Geometry: final body of the model. Coordinates: model frame, mm. A direction names the side the tool comes from. Coordinates: 2 decimals unless noted, no trailing zeros. Loops run counter-clockwise (first coordinate to the right, second up) from the corner with the lowest first, then second, coordinate; pieces in that order, holes last. Notation, with made-up numbers: (-21.5, 36) - (-7.5, 36) arc R20 ccw to (-7.5, 58) - close; hole circle Ø6 at (81.5, -3.75). An arc over 180 degrees is marked (long way). Answer in a Markdown table with one row per item.
from build123d import *

# Parameters (mm, degrees)
SKETCH1_W           = 101.6
SKETCH1_H           = 152.4
BOSS_EXTRUDE1_DEPTH = 3.175
SKETCH2_W           = 3.175
SKETCH2_H           = 12.7
CUT_EXTRUDE1_DEPTH  = 3.175
LPATTERN1_COUNT     = 5
LPATTERN1_PITCH     = 25.4
SKETCH3_W           = 3.175
SKETCH3_H           = 12.7
CUT_EXTRUDE2_DEPTH  = 3.175
LPATTERN2_COUNT     = 4
LPATTERN2_PITCH     = 25.4
SKETCH5_W           = 3.175
SKETCH5_H           = 57.15
CUT_EXTRUDE3_DEPTH  = 3.175
FILLET1_R           = 1.524
BOSS_EXTRUDE2_DEPTH = 3.175
SKETCH7_W           = 25.4
SKETCH7_H           = 95.25
CUT_EXTRUDE4_DEPTH  = 3.175
FILLET2_R           = 12.7


with BuildPart() as part:
    # Sketch1 → Boss-Extrude1 (new body)
    with BuildSketch(Plane(origin=(0, 0, 0), x_dir=(1, 0, 0), z_dir=(0, 1, 0))):
        with Locations((50.8, 76.2)):
            Rectangle(SKETCH1_W, SKETCH1_H)
        Polygon((0, 0), (101.6, -17.91482124), (101.6, 0), align=None)
    extrude(amount=BOSS_EXTRUDE1_DEPTH)

    # Sketch2 → Cut-Extrude1 (cut)
    with BuildSketch(Plane(origin=(0, 3.175, 0), x_dir=(1, 0, 0), z_dir=(0, 1, 0))):
        with Locations((1.5875, 133.35)):
            Rectangle(SKETCH2_W, SKETCH2_H)
    cut_extrude1 = extrude(amount=-CUT_EXTRUDE1_DEPTH, mode=Mode.SUBTRACT)

    # LPattern1: Cut-Extrude1 ×5
    with Locations(*[(0, 0, i * LPATTERN1_PITCH) for i in range(1, LPATTERN1_COUNT)]):
        add(cut_extrude1, mode=Mode.SUBTRACT)

    # Sketch3 → Cut-Extrude2 (cut)
    with BuildSketch(Plane(origin=(0, 3.175, 0), x_dir=(1, 0, 0), z_dir=(0, 1, 0))):
        with Locations((74.6125, 133.35)):
            Rectangle(SKETCH3_W, SKETCH3_H)
    cut_extrude2 = extrude(amount=-CUT_EXTRUDE2_DEPTH, mode=Mode.SUBTRACT)

    # LPattern2: Cut-Extrude2 ×4
    with Locations(*[(0, 0, i * LPATTERN2_PITCH) for i in range(1, LPATTERN2_COUNT)]):
        add(cut_extrude2, mode=Mode.SUBTRACT)

    # Sketch5 → Cut-Extrude3 (cut)
    with BuildSketch(Plane(origin=(0, 3.175, 0), x_dir=(1, 0, 0), z_dir=(0, 1, 0))):
        with Locations((33.3375, 10.66017876)):
            Rectangle(SKETCH5_W, SKETCH5_H)
        with Locations((90.4875, 10.66017876)):
            Rectangle(SKETCH5_W, SKETCH5_H)
    extrude(amount=-CUT_EXTRUDE3_DEPTH, mode=Mode.SUBTRACT)

    # Fillet1
    fillet1_edges = [part.edges().sort_by_distance(p)[0] for p in [
        (34.925, 1.5875, -39.23517876),
        (31.75, 1.5875, -39.23517876),
        (92.075, 1.5875, -39.23517876),
        (88.9, 1.5875, -39.23517876),
    ]]
    fillet(fillet1_edges, radius=FILLET1_R)

    # Sketch6 → Boss-Extrude2 (add)
    with BuildSketch(Plane(origin=(0, 3.175, 0), x_dir=(1, 0, 0), z_dir=(0, 1, 0))):
        Polygon((34.925, -6.158219801), (43.30472917, -7.635792145), (42.753396206, -10.762556761), (34.373667036, -9.284984417), align=None)
        Polygon((55.811787634, -9.841124001), (80.82590456, -14.251787714), (80.274571596, -17.37855233), (55.26045467, -12.967888617), align=None)
    extrude(amount=-BOSS_EXTRUDE2_DEPTH)

    # Sketch7 → Cut-Extrude4 (cut)
    with BuildSketch(Plane(origin=(0, 3.175, 0), x_dir=(1, 0, 0), z_dir=(0, 1, 0))):
        with Locations((22.225, 98.425)):
            Rectangle(SKETCH7_W, SKETCH7_H)
        with Locations((53.975, 98.425)):
            Rectangle(SKETCH7_W, SKETCH7_H)
    extrude(amount=-CUT_EXTRUDE4_DEPTH, mode=Mode.SUBTRACT)

    # Fillet2
    fillet2_edges = [part.edges().sort_by_distance(p)[0] for p in [
        (66.675, 1.5875, -146.05),
        (34.925, 1.5875, -146.05),
        (41.275, 1.5875, -146.05),
        (9.525, 1.5875, -146.05),
        (34.925, 1.5875, -50.8),
        (41.275, 1.5875, -50.8),
        (66.675, 1.5875, -50.8),
        (9.525, 1.5875, -50.8),
    ]]
    fillet(fillet2_edges, radius=FILLET2_R - 0.0001)  # a hair under: the kernel refuses the full size


solid = part.part
(1) Cut plane C-C on z = -70. Output: boundary loops of the cut face in (x, y) (3 decimals).
Verdict:
| item | result |
|---|---|
| outline | (0, 0) - (9.525, 0) - (9.525, 3.175) - (0, 3.175) - close; (34.925, 0) - (41.275, 0) - (41.275, 3.175) - (34.925, 3.175) - close; (66.675, 0) - (101.6, 0) - (101.6, 3.175) - (66.675, 3.175) - close |
(2) Cut plane A-A on z = -23.5. Output: boundary loops of the cut face in (x, y) (3 decimals), then the cut area to 3 significant figures.
Verdict:
| item | result |
|---|---|
| outline | (0, 0) - (31.75, 0) - (31.75, 3.175) - (0, 3.175) - close; (34.925, 0) - (88.9, 0) - (88.9, 3.175) - (34.925, 3.175) - close; (92.075, 0) - (101.6, 0) - (101.6, 3.175) - (92.075, 3.175) - close |
| area | 302 mm² |
(3) Cut plane B-B on x = 26.5. Output: boundary loops of the cut face in (y, z) (3 decimals), then the cut area to 3 significant figures.
Verdict:
| item | result |
|---|---|
| outline | (0, -152.4) - (3.175, -152.4) - (3.175, -145.309) - (0, -145.309) - close; (0, -51.541) - (3.175, -51.541) - (3.175, 4.673) - (0, 4.673) - close |
| area | 201 mm² |
(4) Access query for faces 1 (the face through (75, 2, -127)), 2 (the face through (43.033, 1.61, 9.177)), 3 (the face through (67.943, 1.61, 15.204)), 4 (the face through (2, 2, -38.1)). Directions: +Z, -Z, +X, -X, +Y, -Y. A direction counts if a zero-diameter tool reaches every point of the face in a straight line with its end or side. Return the directions, or none.
Verdict:
| item | result |
|---|---|
| face 1 | +Y, -Y |
| face 2 | +Z, +Y, -Y |
| face 3 | +Z, -X, +Y, -Y |
| face 4 | -X, +Y, -Y |
(5) First-contact query: pin 1 Ø1 at (x, y) = (1, 1) entering from +Z; pin 2 Ø1 at (y, z) = (2, -58) entering from -X (3 decimals); pin 3 Ø6 at (x, z) = (47, -85) entering from -Y. Flat tips, straight axial feed; report the tip coordinate or a pass-through.
Verdict:
| item | result |
|---|---|
| pin 1 | stops at z = 0.26 |
| pin 2 | stops at x = 3.175 |
| pin 3 | passes through |
(6) Ray query, probe 1 along X at (y, z) = (1, -2.5) (3 decimals); probe 2 along X at (y, z) = (2.45, -104) (3 decimals); probe 3 along X at (y, z) = (0.2, -119.5) (3 decimals). Return the intervals inside material, ascending.
Verdict:
| item | result |
|---|---|
| probe 1 | x = 0 to 31.75, 34.925 to 88.9, 92.075 to 101.6 |
| probe 2 | x = 3.175 to 9.525, 34.925 to 41.275, 66.675 to 73.025, 76.2 to 101.6 |
| probe 3 | x = 0 to 9.525, 34.925 to 41.275, 66.675 to 101.6 |
(7) Pull-direction query (Z, two-part tool) for faces 5 (the face through (2, 2, -63.5)), 6 (the face through (80.554, 1.61, 15.793)), 7 (the face through (0, 2, -121)); classes: pulls with the +Z half, pulls with the -Z half, needs draft (parallel to the pull), parting line crosses it, or undercut.
Verdict:
| item | result |
|---|---|
| face 5 | undercut |
| face 6 | pulls with the +Z half |
| face 7 | needs draft |
(8) Cut plane D-D on y = 2.5. State how many separate pieces and enclosed holes the cut face has, then the cut area to 3 significant figures.
Verdict:
| item | result |
|---|---|
| separate pieces | 1 |
| enclosed holes | 6 |
| area | 11,300 mm² |
